Input: dimensioned drawing with shaded views. Units: mm. Origin: part minimum x, y, z. Coordinates: 2 decimals unless noted, no trailing zeros. Order: outer loops, then holes, each group sorted by start corner. A loop starts at its lowest first (then second) coordinate and runs counter-clockwise, first axis right, second up. Notation, with made-up numbers: (18, 87) - (69, 87) arc R11 ccw to (69, 97) - close; hole circle Ø10 at (33, 43). An arc over 180 degrees is marked (long way). One line per question, with ' | ' between items. Start each with the question number.
(1) Section C-C (z = 4.5). Count the separate pieces of the cut face and the enclosed holes in it, then the cut area to 3 significant figures.
(2) Line query: line 1 along X through (y, z) = (118, 4.5); line 2 along X through (y, z) = (89, 5.25); line 3 along Z through (x, y) = (19, 2). Output: solid intervals per line, ascending.
(3) Section A-A (x = 121.5). Return the cut outline in (y, z).
(4) Contact query for flat-ended pins moving along their axis: P1, Ø0.9, axis at x = 171.5, z = 4, coming from the +Y side; P2, Ø2.5, axis at x = 4.5, y = 60, coming from the -Z side. Output: stop coordinate, or through.
(5) Section B-B (y = 48.5). Return the cut outline in (x, z), then the cut area to 4 significant figures.
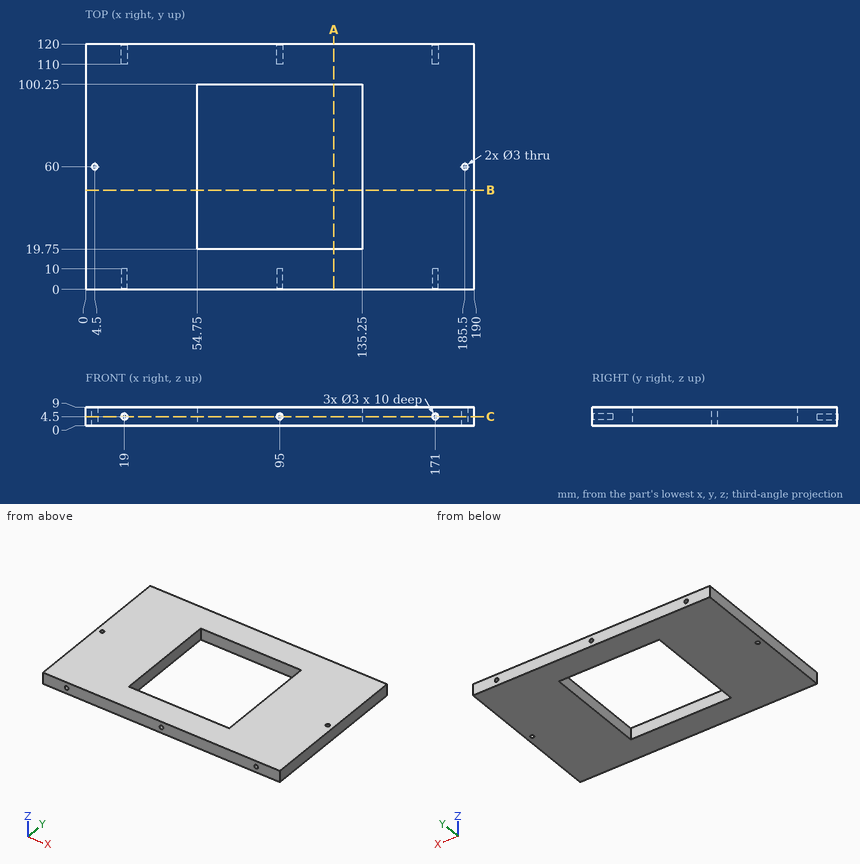
Response values:
1) separate pieces: 1 | enclosed holes: 3 | area: 16,100 mm²
2) line 1: x = 0 to 17.5, 20.5 to 93.5, 96.5 to 169.5, 172.5 to 190 | line 2: x = 0 to 54.75, 135.25 to 190 | line 3: z = 0 to 3, 6 to 9
3) outline: (0, 0) - (19.75, 0) - (19.75, 9) - (0, 9) - close; (100.25, 0) - (120, 0) - (120, 9) - (100.25, 9) - close
4) P1: stops at y = 110 | P2: passes through
5) outline: (0, 0) - (54.75, 0) - (54.75, 9) - (0, 9) - close; (135.25, 0) - (190, 0) - (190, 9) - (135.25, 9) - close | area: 985.5 mm²
